```python
from build123d import *

# Parameters (mm, degrees)
PAD009_DEPTH    = 57
SKETCH031_R     = 3.5
POCKET005_DEPTH = 7.5
THICKNESS_T     = -2.5
SKETCH032_R     = 1.5
PAD010_DEPTH    = 2.5
SKETCH033_R     = 2.4
PAD011_DEPTH    = 33
PAD012_DEPTH    = 2.5
PAD013_DEPTH    = 5
PAD014_DEPTH    = 5


with BuildPart() as part:
    # Sketch030 → Pad009 (new body)
    with BuildSketch(Plane(origin=(0, 0, 0), x_dir=(0, -1, 0), z_dir=(-1, 0, 0))):
        with BuildLine():
            Line((-56.9812455945, -19.1666932293), (-85.3849313131, 115.5624248602))
            ThreePointArc((-76.5785062018, 126.4190014838), (-83.5681124, 123.0886932914), (-85.3849313131, 115.5624248602))
            Line((-76.5785062018, 126.4190014838), (-56.5746674209, 126.4190014838))
            ThreePointArc((-56.5746674209, 126.4190014838), (-49.173982549, 110.8865432655), (-32.4489415907, 106.8491679032))
            Line((-32.4489415907, 106.8491679032), (-8.0566616429, -8.8523786537))
            Line((-8.0566616429, -8.8523786537), (-56.9812455945, -19.1666932293))
        make_face()
    extrude(amount=PAD009_DEPTH)

    # Sketch031 → Pocket005 (cut)
    with BuildSketch(Plane.YZ):
        with Locations((40.4092527683, 49.4266176238)):
            Circle(SKETCH031_R)
        with Locations((67.6714613195, 115.017708736)):
            Circle(SKETCH031_R)
    extrude(amount=-POCKET005_DEPTH, mode=Mode.SUBTRACT)

    # Thickness
    thickness_openings = [part.faces().sort_by_distance(p)[0] for p in [
        (-57, 47.670985, 52.690427),
    ]]
    offset(amount=THICKNESS_T, openings=thickness_openings)

    # Sketch032 → Pad010 (join)
    with BuildSketch(Plane(origin=(0, 0, 0), x_dir=(0, -1, 0), z_dir=(-1, 0, 0))):
        with BuildLine():
            ThreePointArc((-76.5785062018, 126.4190014838), (-83.5681124, 123.0886932914), (-85.3849313131, 115.5624248602))
            Line((-85.3849313131, 115.5624248602), (-82.6454361548, 102.5679927173))
            ThreePointArc((-82.6454361548, 102.5679927173), (-84.5605229517, 106.5001513818), (-88.1031081238, 109.0652087887))
            ThreePointArc((-84.7543549815, 126.4190014838), (-93.5913265854, 119.1242677012), (-88.1031081238, 109.0652087887))
            Line((-84.7543549815, 126.4190014838), (-76.5785062018, 126.4190014838))
        make_face()
        with Locations((-89.5482969155, 118.3440861841)):
            Circle(SKETCH032_R, mode=Mode.SUBTRACT)
        with BuildLine():
            ThreePointArc((-14.6548301134, 103.446667091), (-17.6820502047, 107.8670148106), (-22.9482759072, 108.8521048036))
            Line((-32.4489415907, 106.8491679032), (-22.9482759072, 108.8521048036))
            Line((-32.4489415907, 106.8491679032), (-29.5104359602, 92.9107559656))
            Line((-29.5104359602, 92.9107559656), (-20.0097702767, 94.9136928661))
            ThreePointArc((-11.7163244829, 89.5082551534), (-14.7435445743, 93.928602873), (-20.0097702767, 94.9136928661))
            Line((-14.6548301134, 103.446667091), (-11.7163244829, 89.5082551534))
        make_face()
        with Locations((-21.5042718666, 102.0026630504)):
            Circle(SKETCH032_R, mode=Mode.SUBTRACT)
        with BuildLine():
            ThreePointArc((-15.3271793951, 25.6343585435), (-12.2999593038, 21.2140108239), (-7.0337336013, 20.2289208309))
            Line((-7.0337336013, 20.2289208309), (-4.382509671, 20.7878536908))
            ThreePointArc((3.9109361228, 15.3824159782), (0.8837160314, 19.8027636978), (-4.382509671, 20.7878536908))
            Line((3.9109361228, 15.3824159782), (6.8494417532, 1.4440040406))
            ThreePointArc((6.8494417532, 1.4440040406), (3.8222216619, 5.8643517602), (-1.4440040406, 6.8494417532))
            Line((-10.9446697241, 4.8465048527), (-1.4440040406, 6.8494417532))
            Line((-15.3271793951, 25.6343585435), (-10.9446697241, 4.8465048527))
        make_face()
        with Locations((-2.9385056304, 13.9384119376)):
            Circle(SKETCH032_R, mode=Mode.SUBTRACT)
        with BuildLine():
            ThreePointArc((-63.9746959939, -5.3847157517), (-65.7656124274, -14.9588361058), (-56.9812455945, -19.1666932293))
            Line((-61.489922629, 2.2196186258), (-56.9812455945, -19.1666932293))
            ThreePointArc((-63.9746959939, -5.3847157517), (-61.7135216838, -1.9154450712), (-61.489922629, 2.2196186258))
        make_face()
        with Locations((-62.0562568032, -12.0607618174)):
            Circle(SKETCH032_R, mode=Mode.SUBTRACT)
    extrude(amount=PAD010_DEPTH)

    # Sketch033 → Pad011 (join)
    with BuildSketch(Plane(origin=(0, 0, 0), x_dir=(0, -1, 0), z_dir=(-1, 0, 0))):
        with BuildLine():
            Line((-29.5104359602, 92.9107559656), (-20.0097702767, 94.9136928661))
            ThreePointArc((-17.1217621955, 81.2148093596), (-11.7163244829, 89.5082551534), (-20.0097702767, 94.9136928661))
            Line((-17.1217621955, 81.2148093596), (-26.6224278791, 79.2118724591))
            Line((-29.5104359602, 92.9107559656), (-26.6224278791, 79.2118724591))
        make_face()
        with Locations((-18.5657662361, 88.0642511128)):
            Circle(SKETCH033_R, mode=Mode.SUBTRACT)
        with BuildLine():
            Line((-10.9446697241, 4.8465048527), (-1.4440040406, 6.8494417532))
            ThreePointArc((1.4440040406, -6.8494417532), (6.8494417532, 1.4440040406), (-1.4440040406, 6.8494417532))
            Line((1.4440040406, -6.8494417532), (-8.0566616429, -8.8523786537))
            Line((-10.9446697241, 4.8465048527), (-8.0566616429, -8.8523786537))
        make_face()
        Circle(SKETCH033_R, mode=Mode.SUBTRACT)
    extrude(amount=PAD011_DEPTH)

    # Sketch035 (on Face2 of Pad011) → Pad012 (join)
    with BuildSketch(Plane(origin=(-2.5, 0, 0), x_dir=(0, -1, 0), z_dir=(-1, 0, 0))):
        with BuildLine():
            Line((-47.3206478613, -14.5750866), (-55.0507321257, -16.204748303))
            Line((-55.0507321257, -16.204748303), (-82.9387021155, 116.0781405889))
            ThreePointArc((-76.5785062018, 123.9190014838), (-81.6265551227, 121.5137789004), (-82.9387021155, 116.0781405889))
            Line((-76.5785062018, 123.9190014838), (-76.5180671542, 123.9190014838))
            Line((-76.5180671542, 123.9190014838), (-47.3206478613, -14.5750866))
        make_face()
        Polygon((-77.2796270866, 112.9884644786), (-79.1387612768, 112.5965205247), (-53.7655474207, -7.7579559962), (-51.9064132305, -7.3660120423), align=None, mode=Mode.SUBTRACT)
    extrude(amount=PAD012_DEPTH)

    # Sketch037 (on Face2 of Pad011) → Pad013 (join)
    with BuildSketch(Plane(origin=(-2.5, 0, 0), x_dir=(0, -1, 0), z_dir=(-1, 0, 0))):
        Polygon((-20.1983465416, 36.621014532), (-27.5370341343, 35.0738673456), (-30.3218990697, 48.2835050126), (-22.983211477, 49.8306521989), align=None)
        Polygon((-39.089066459, 89.8694013714), (-31.7503788663, 91.4165485578), (-28.9655139309, 78.2069108908), (-36.3042015236, 76.6597637045), align=None)
    extrude(amount=PAD013_DEPTH)

    # Sketch036 (on Face2 of Pad011) → Pad014 (join)
    with BuildSketch(Plane(origin=(-7.5, 0, 0), x_dir=(0, -1, 0), z_dir=(-1, 0, 0))):
        Polygon((-20.1983465416, 36.621014532), (-27.5370341343, 35.0738673456), (-30.3218990697, 48.2835050126), (-27.3864240326, 48.9023638871), (-25.6329905548, 40.5851846153), (-24.1652530362, 40.8946140526), (-25.9186865141, 49.2117933244), (-22.983211477, 49.8306521989), align=None)
        Polygon((-39.089066459, 89.8694013714), (-31.7503788663, 91.4165485578), (-28.9655139309, 78.2069108908), (-31.900988968, 77.5880520163), (-33.6544224458, 85.9052312881), (-35.1221599644, 85.5958018508), (-33.3687264865, 77.278622579), (-36.3042015236, 76.6597637045), align=None)
    extrude(amount=PAD014_DEPTH)


solid = part.part
```
Part model, mm, in its own coordinate system. A direction names the side the tool comes from. Give positions to 0.01 mm unless a question says otherwise; leave off trailing zeros. Order: outer loops, then holes, each group sorted by start corner. A loop starts at its lowest first (then second) coordinate and runs counter-clockwise, first axis right, second up. Notation, with made-up numbers: (76.5, 28.25) - (112.5, 28.25) arc R13 cw to (112.5, 37.25) - close; hole circle Ø7 at (86, 2). An arc over 180 degrees is marked (long way). Use one line per item in the form item = value.
Item 1: Two-plate mould, pull along Z, no slides. Class faces 1 (the face through (-2.5, 43, 56)), 2 (the face through (-1.232, 17.618, 107.825)): released by +Z, released by -Z, zero draft, split by the parting line, or undercut.
Solution:
face_1 = undercut
face_2 = released by +Z
Item 2: Pin check, flat tips, straight feed: pin 1 Ø4 at (y, z) = (37.5, 70) entering from +X; pin 2 Ø1 at (x, y) = (-22.5, 10) entering from +Z; pin 3 Ø6 at (x, z) = (-9.5, 52) entering from -Y; pin 4 Ø3.5 at (y, z) = (89.55, 118.34) entering from -X. Stop position of each tip, or through.
Solution:
pin_1 = 0
pin_2 = 5.15
pin_3 = 20.25
pin_4 = -2.5
Item 3: Which spindle directions (+Z, -Z, +X, -X, +Y, -Y) get a long thin tool onto all of the face, cutting with end or side? Do faces 3 (the face through (-1.232, 3.264, 12.474)), 4 (the face through (-9.96, 26.52, 44.8)). Say none if no direction does.
Solution:
face_3 = +X, -X
face_4 = -X
Item 4: Probe probe 1 along Y at (x, z) = (-4.5, 60); probe 2 along Z at (x, y) = (-8.5, 40.5); probe 3 along X at (y, z) = (50, 89.5). List the from-to ranges inside material, lowest first. Write a range as from..to.
Solution:
probe_1 = 22.57..25.13, 63.04..66.11, 68.05..73.67
probe_2 = -15.69..-13.14, 43.64..55.22, 104.26..106.81
probe_3 = -2.5..0
Item 5: Slice it at A-A on x = -38. Give the cut face in (y, z), and give its area (3 significant figures).
Solution:
outline = (8.06, -8.85) - (56.98, -19.17) - (85.38, 115.56) arc R9 ccw to (76.58, 126.42) - (56.57, 126.42) arc R20 cw to (32.45, 106.85) - close; hole (11.02, -6.92) - (55.05, -16.2) - (82.94, 116.08) arc R6.5 ccw to (76.58, 123.92) - (58.94, 123.92) arc R22.5 cw to (34.41, 104.02) - close
area = 919 mm2
